Print and shaded views of the part. All mm, measured from the part's lowest x, y and z. Give positions to 0.01 mm unless a question says otherwise; leave off trailing zeros. Order: outer loops, then holes, each group sorted by start corner. A loop starts at its lowest first (then second) coordinate and runs counter-clockwise, first axis right, second up. Notation, with made-up numbers: (-25.5, 32.5) - (-6.5, 32.5) arc R30 ccw to (-6.5, 58.5) - close; hole circle Ø6 at (60.25, 7). An arc over 180 degrees is marked (long way). Answer in a Markdown table with one row per item.
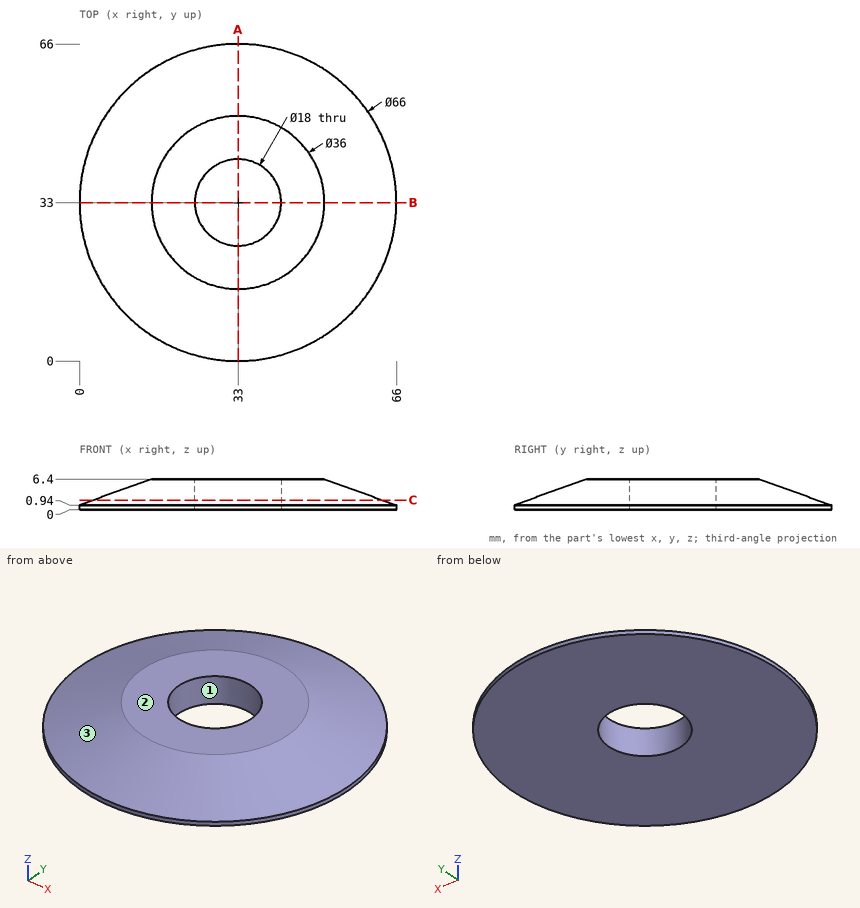
1. Cut at C-C on z = 2. Write the cut outline in (x, y).
Check result:
| item | result |
|---|---|
| outline | circle Ø60.18 at (33, 33); hole circle Ø18 at (33, 33) |
2. Probe line 1 (X direction, y = 40.5, z = 0.5) (1 decimal); line 2 (Z direction, x = 61, y = 33.5); line 3 (Z direction, x = 50.5, y = 44). List the from-to ranges inside material, lowest first.
Check result:
| item | result |
|---|---|
| line 1 | x = 0.9 to 28, 38 to 65.1 |
| line 2 | z = 0 to 2.76 |
| line 3 | z = 0 to 5.43 |
3. Cut at A-A on x = 33. Write the cut outline in (y, z), and give its area (3 significant figures).
Check result:
| item | result |
|---|---|
| outline | (0, 0) - (24, 0) - (24, 6.4) - (15, 6.4) - (0, 0.94) - close; (42, 0) - (66, 0) - (66, 0.94) - (51, 6.4) - (42, 6.4) - close |
| area | 225 mm² |
4. Two-plate mould, pull along Y, no slides. Class the marked faces 1, 2 and 3: +Y half, -Y half, draft (parallel to the pull), parting line (faces both ways), or undercut.
Check result:
| item | result |
|---|---|
| face 1 | undercut |
| face 2 | draft |
| face 3 | parting line |
